Geometry: final body of the model. Coordinates: model frame, mm. Face numbers are marked on the shaded views. A direction names the side the tool comes from. Coordinates: 2 decimals unless noted, no trailing zeros. Order: outer loops, then holes, each group sorted by start corner. A loop starts at its lowest first (then second) coordinate and runs counter-clockwise, first axis right, second up. Notation, with made-up numbers: (58.25, 64.25) - (91.25, 64.25) arc R22 ccw to (91.25, 82.25) - close; hole circle Ø9 at (42, 43.25). An arc over 180 degrees is marked (long way). Use one line per item in the form item = value. Start each with the question number.
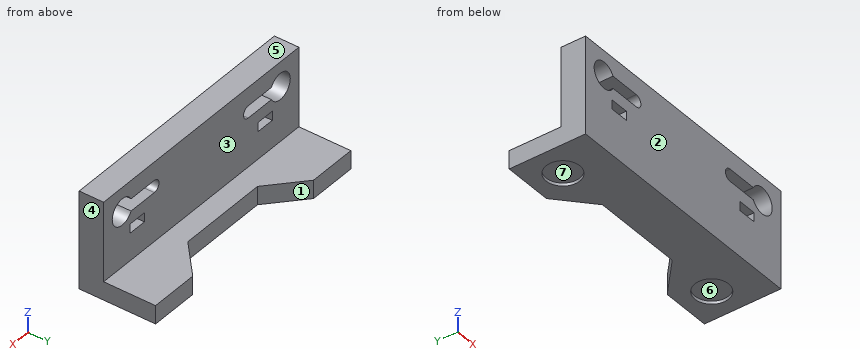
```python
from build123d import *

# Parameters (mm, degrees)
SKETCH2_W           = 84
SKETCH2_H           = 32
SKETCH2_W_2         = 6.1
SKETCH2_H_2         = 3
BOSS_EXTRUDE2_DEPTH = 8
BOSS_EXTRUDE3_DEPTH = 6
SKETCH4_R           = 5.5
CUT_EXTRUDE1_DEPTH  = 1


with BuildPart() as part:
    # Sketch2 → Boss-Extrude2 (new body)
    with BuildSketch(Plane(origin=(0, 0, 0), x_dir=(1, 0, 0), z_dir=(0, 1, 0))):
        with Locations((0, 16)):
            Rectangle(SKETCH2_W, SKETCH2_H)
        with BuildLine():
            ThreePointArc((20.193426738, 10), (18.193426738, 8), (20.193426738, 6))
            Line((20.193426738, 6), (30.193426738, 6))
            ThreePointArc((30.193426738, 6), (38.3, 8), (30.193426738, 10))
            Line((30.193426738, 10), (20.193426738, 10))
        make_face(mode=Mode.SUBTRACT)
        with BuildLine():
            ThreePointArc((-30.193426738, 10), (-38.3, 8), (-30.193426738, 6))
            Line((-30.193426738, 6), (-20.193426738, 6))
            ThreePointArc((-20.193426738, 6), (-18.193426738, 8), (-20.193426738, 10))
            Line((-20.193426738, 10), (-30.193426738, 10))
        make_face(mode=Mode.SUBTRACT)
        with Locations((27.5, 15.5)):
            Rectangle(SKETCH2_W_2, SKETCH2_H_2, mode=Mode.SUBTRACT)
        with Locations((-27.5, 15.5)):
            Rectangle(SKETCH2_W_2, SKETCH2_H_2, mode=Mode.SUBTRACT)
    extrude(amount=BOSS_EXTRUDE2_DEPTH)

    # Sketch3 → Boss-Extrude3 (add)
    with BuildSketch(Plane(origin=(0, 0, -32), x_dir=(-1, 0, 0), z_dir=(0, 0, -1))):
        Polygon((-42, 8), (-42, 25), (-26, 25), (-15, 15), (15, 15), (26, 25), (42, 25), (42, 8), align=None)
    extrude(amount=-BOSS_EXTRUDE3_DEPTH)

    # Sketch4 → Cut-Extrude1 (cut)
    with BuildSketch(Plane(origin=(0, 0, -32), x_dir=(-1, 0, 0), z_dir=(0, 0, -1))):
        with Locations((32, 15)):
            Circle(SKETCH4_R)
        with Locations(Location((-32, 15, 0), (0, 0, 180))):
            Circle(SKETCH4_R)
    extrude(amount=-CUT_EXTRUDE1_DEPTH, mode=Mode.SUBTRACT)


solid = part.part
```
(1) Material intervals for L1, parallel to Y at x = 32, z = -31.5; L2, parallel to X at y = 5.5, z = -14.5; L3, parallel to Z at x = -34, y = 4.5, sorted ascending. Write a range as from..to.
(2) Draft query along X for the marked faces 4, 5, 6 and 7. Return one class per face: released by +X, released by -X, zero draft, split by the parting line, or undercut.
(3) Contact query for flat-ended pins moving along their axis: pin 1 Ø4 at (x, y) = (25, 5) entering from +Z; pin 2 Ø12 at (x, z) = (-23, -5.5) entering from +Y; pin 3 Ø3.5 at (x, y) = (31, 15.5) entering from -Z; pin 4 Ø6.5 at (x, y) = (32, 15) entering from +Z. Output: stop coordinate, or through.
(4) Set-up query: the marked faces 1, 2 and 3. Return all of +Z, -Z, +X, -X, +Y, -Y with unobstructed straight access to the full face (end or side cutting, diameter ignored); none if empty.
(5) Cut plane B-B on y = 2.5. Return the cut outline in (x, z), plus the area to 3 significant figures.
(6) Cut plane C-C on x = -35. Return the cut outline in (y, z), plus the area to 3 significant figures.
(7) Cut plane D-D on z = -15. Return the cut outline in (x, y).
(8) Cut plane A-A on z = -8. Return the cut outline in (x, y), plus the area to 3 significant figures.
Check sheet entries:
q1.L1 = 0..9.5, 20.5..25
q1.L2 = -42..-30.55, -24.45..24.45, 30.55..42
q1.L3 = -32..-12.3, -3.7..0
q2.face_4 = released by +X
q2.face_5 = zero draft
q2.face_6 = undercut
q2.face_7 = undercut
q3.pin_1 = 0
q3.pin_2 = 8
q3.pin_3 = -31
q3.pin_4 = -26
q4.face_1 = +Z, -Z, +Y
q4.face_2 = +Z, -Z, +X, -X, -Y
q4.face_3 = +Z, +X, -X, +Y
q5.outline = (-42, -32) - (42, -32) - (42, 0) - (-42, 0) - close; hole (-30.55, -17) - (-24.45, -17) - (-24.45, -14) - (-30.55, -14) - close; hole (-30.19, -10) - (-20.19, -10) arc R2 ccw to (-20.19, -6) - (-30.19, -6) arc R4.3 ccw (long way) to start; hole (20.19, -10) - (30.19, -10) arc R4.3 ccw (long way) to (30.19, -6) - (20.19, -6) arc R2 ccw to start; hole (24.45, -17) - (30.55, -17) - (30.55, -14) - (24.45, -14) - close
q5.area = 2,450 mm^2
q6.outline = (0, -32) - (10.39, -32) - (10.39, -31) - (19.61, -31) - (19.61, -32) - (25, -32) - (25, -26) - (8, -26) - (8, -12.18) - (0, -12.18) - close; (0, -3.82) - (8, -3.82) - (8, 0) - (0, 0) - close
q6.area = 282 mm^2
q7.outline = (-42, 0) - (-30.55, 0) - (-30.55, 8) - (-42, 8) - close; (-24.45, 0) - (24.45, 0) - (24.45, 8) - (-24.45, 8) - close; (30.55, 0) - (42, 0) - (42, 8) - (30.55, 8) - close
q8.outline = (-42, 0) - (-38.3, 0) - (-38.3, 8) - (-42, 8) - close; (-18.19, 0) - (18.19, 0) - (18.19, 8) - (-18.19, 8) - close; (38.3, 0) - (42, 0) - (42, 8) - (38.3, 8) - close
q8.area = 350 mm^2
